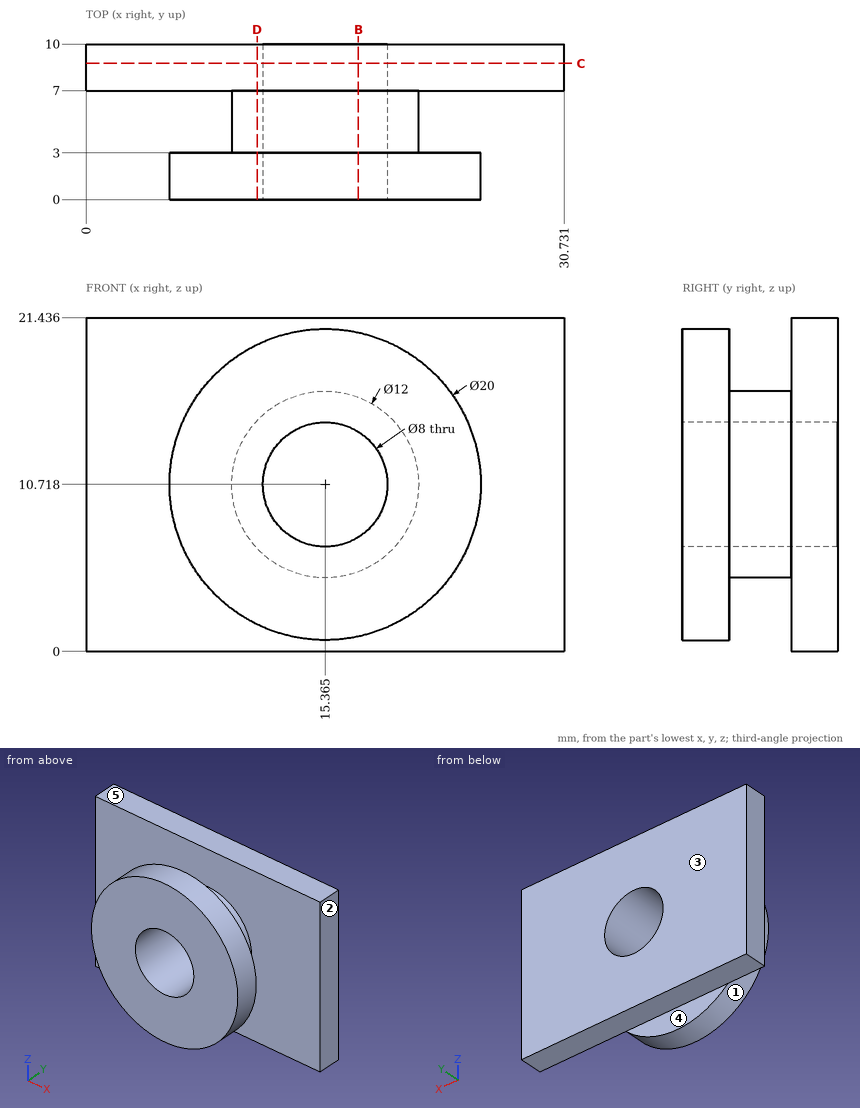
Can you work these out from the drawing? Everything is in mm from the part's minimum corner. A direction names the side the tool comes from. Coordinates: 2 decimals unless noted, no trailing zeros. Loops run counter-clockwise (first coordinate to the right, second up) from the corner with the lowest first, then second, coordinate; pieces in that order, holes last.
1. Imagine slicing it at C-C, the plane y = 8.75. Please give me the cut outline in (x, z) (1 decimal).
2. If we mould it in two halves opening along Y, with no side actions, what happens to the marked faces 3, 4 and 5? For each: pulls with the +Y half, pulls with the -Y half, needs draft (parallel to the pull), parting line crosses it, or undercut.
3. I need wall thicknesses on L1, parallel to Y at x = 15.5, z = 18.5; L2, parallel to Z at x = 16, y = 9 (1 decimal); L3, parallel to X at y = 6.75, z = 8.75 (1 decimal). Which ranges of each line are inside material? Lowest first, please.
4. Imagine slicing it at D-D, the plane x = 11. Please give me the cut outline in (y, z) (1 decimal).
5. For the marked faces 1 and 2, which set-ups out of +Z, -Z, +X, -X, +Y, -Y let a thin tool reach every point of the face, with its end or its side?
6. Imagine slicing it at B-B, the plane x = 17.5. Please give me the cut outline in (y, z) (1 decimal), and give its area (3 significant figures).
7. For P1, Ø6, axis at x = 18, z = 12, coming from the +Y side; P2, Ø2, axis at y = 5.5, z = 13.5, coming from the -X side; P3, Ø1.5, axis at x = 7, y = 3, coming from the +Z side, each with a flat end and sliding along its axis, tell me the tip position at first contact or that it passes through.
Taken from the geometry:
1. outline: (0, 0) - (30.7, 0) - (30.7, 21.4) - (0, 21.4) - close; hole circle Ø8 at (15.4, 10.7)
2. face 3: pulls with the +Y half
2. face 4: undercut
2. face 5: needs draft
3. L1: y = 0 to 3, 7 to 10
3. L2: z = 0 to 6.8, 14.7 to 21.4
3. L3: x = 9.7 to 11.9, 18.8 to 21
4. outline: (0, 1.7) - (3, 1.7) - (3, 6.6) - (7, 6.6) - (7, 0) - (10, 0) - (10, 21.4) - (7, 21.4) - (7, 14.8) - (3, 14.8) - (3, 19.7) - (0, 19.7) - close
5. face 1: -Y
5. face 2: +Z, -Z, +X, +Y, -Y
6. outline: (0, 0.9) - (3, 0.9) - (3, 5.1) - (7, 5.1) - (7, 0) - (10, 0) - (10, 7.3) - (0, 7.3) - close; (0, 14.1) - (10, 14.1) - (10, 21.4) - (7, 21.4) - (7, 16.3) - (3, 16.3) - (3, 20.5) - (0, 20.5) - close
6. area: 100 mm2
7. P1: stops at y = 10
7. P2: stops at x = 9.64
7. P3: stops at z = 17.2
